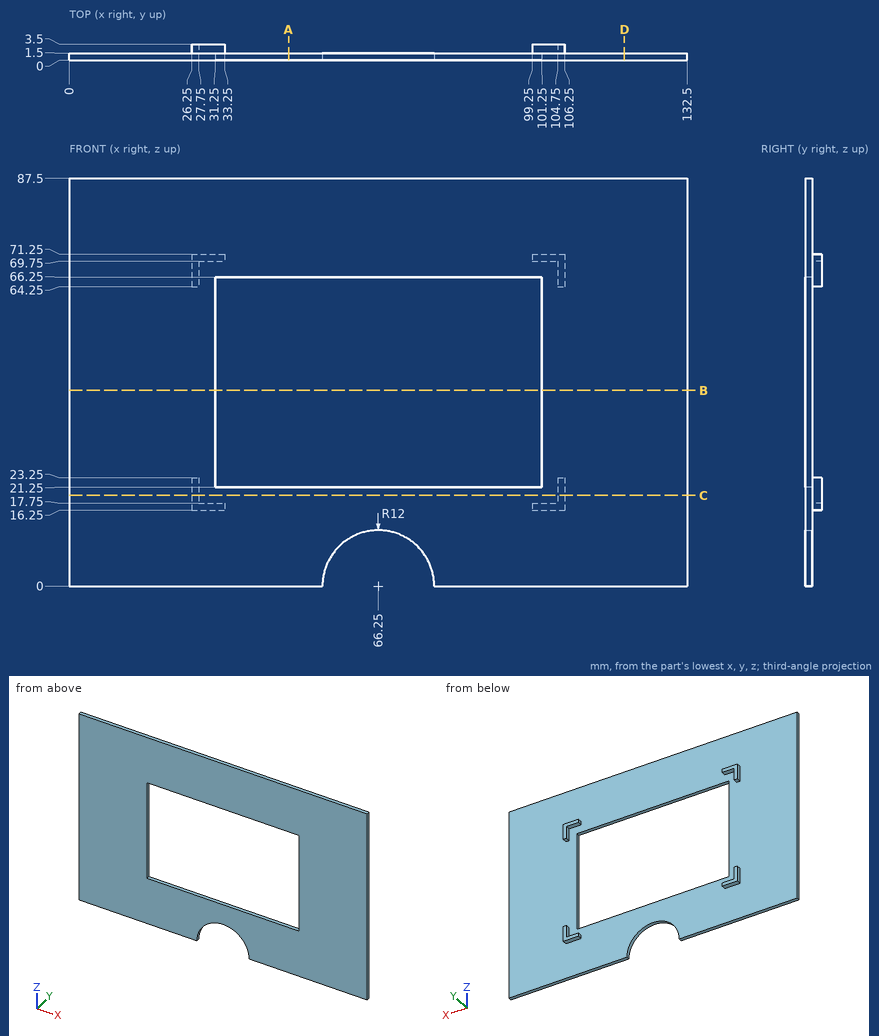
Geometry check sheet. Reference: drawing and pictorial views, mm from the part's lowest x, y, z. Give positions to 0.01 mm unless a question says otherwise; leave off trailing zeros. Loops run counter-clockwise (first coordinate to the right, second up) from the corner with the lowest first, then second, coordinate; pieces in that order, holes last. Notation, with made-up numbers: (55, 41) - (84, 41) arc R23 cw to (84, 79) - close; hole circle Ø7 at (76, -27). An arc over 180 degrees is marked (long way). One line per question, with ' | ' between items. Start each with the question number.
1. Cross-section at B-B, the plane z = 42. Enter the section's corners in (x, y), plus the area to 4 significant figures.
2. Cross-section at D-D, the plane x = 119. Enter the section's corners in (y, z).
3. Material ranges on line 1 along Z through (x, y) = (94, 0.3); line 2 along Z through (x, y) = (102, 1.7); line 3 along X through (y, z) = (0.35, 53.5), recorded low to high. Write a range as [from, to].
4. Gauge pin test, flat ends, axial feed: pin 1 Ø1.6 at (x, y) = (105.5, 2) entering from +Z; pin 2 Ø1.2 at (x, y) = (105.5, 2.5) entering from -Z; pin 3 Ø0.6 at (y, z) = (3, 21) entering from -X; pin 4 Ø1 at (y, z) = (3, 66) entering from +X. Record the tip position at first contact, or that the pin passes through.
5. Cross-section at C-C, the plane z = 19.5. Enter the section's corners in (x, y), plus the area to 3 significant figures.
6. Cross-section at A-A, the plane x = 47. Enter the section's corners in (y, z), plus the area to 4 significant figures.
Check result:
1) outline: (0, 0) - (31.25, 0) - (31.25, 1.5) - (0, 1.5) - close; (101.25, 0) - (132.5, 0) - (132.5, 1.5) - (101.25, 1.5) - close | area: 93.75 mm2
2) outline: (0, 0) - (1.5, 0) - (1.5, 87.5) - (0, 87.5) - close
3) line 1: z = [0, 21.25], [66.25, 87.5] | line 2: z = [16.25, 17.75], [69.75, 71.25] | line 3: x = [0, 31.25], [101.25, 132.5]
4) pin 1: stops at z = 87.5 | pin 2: stops at z = 16.25 | pin 3: stops at x = 26.25 | pin 4: stops at x = 106.25
5) outline: (0, 0) - (132.5, 0) - (132.5, 1.5) - (106.25, 1.5) - (106.25, 3.5) - (104.75, 3.5) - (104.75, 1.5) - (27.75, 1.5) - (27.75, 3.5) - (26.25, 3.5) - (26.25, 1.5) - (0, 1.5) - close | area: 205 mm2
6) outline: (0, 0) - (1.5, 0) - (1.5, 21.25) - (0, 21.25) - close; (0, 66.25) - (1.5, 66.25) - (1.5, 87.5) - (0, 87.5) - close | area: 63.75 mm2
